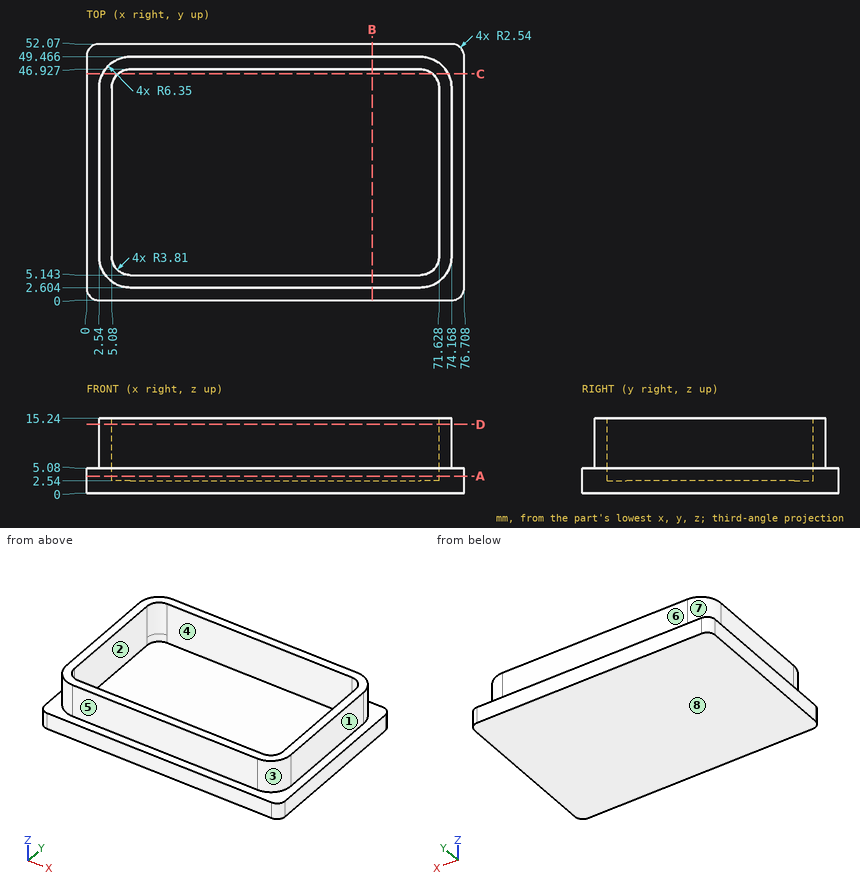
Drawing for the job (mm, zero at the part's lowest x, y, z). A direction names the side the tool comes from. Round coordinates to 2 decimals unless told otherwise and drop trailing zeros. Loops run counter-clockwise (first coordinate to the right, second up) from the corner with the lowest first, then second, coordinate; pieces in that order, holes last. Notation, with made-up numbers: M 11,68.25 L 17,68.25 A17 cw 17,99.25 Z; hole C -10,73 d1. An arc over 180 degrees is marked long. Use a Markdown table: item, result. Add a question column.
(1) Cut at A-A (z = 3.5). Give the cut face in (x, y), and give its area (3 significant figures).
(2) Flat gauge pins, fed straight in: pin 1 (4 mm diameter, centred on x = 20, z = 8.5, fed in from +Y); pin 2 (5 mm diameter, centred on y = 22.5, z = 10.5, fed in from +X); pin 3 (2 mm diameter, centred on x = 65, y = 16, fed in from +Z). Where does each tip first touch, or does it go through?
(3) Cut at B-B (x = 58). Give the cut face in (y, z).
(4) Cut at D-D (z = 14). Give the cut face in (x, y).
(5) Cut at C-C (y = 46). Give the cut face in (x, z) (1 decimal).
(6) Pull direction Y, two halves, no side cores. Call the marked faces 1, 2 and 3: +Y half, -Y half, draft (parallel to the pull), parting line (faces both ways), or undercut.
(7) Which spindle directions (+Z, -Z, +X, -X, +Y, -Y) get a long thin tool onto all of the face, cutting with end or side? Do the marked faces 4, 5, 6, 7 and 8. Say none if no direction does.
(8) Drill centre lines: line 1 (Y direction, x = 30, z = 5.75); line 2 (X direction, y = 25, z = 12.5); line 3 (X direction, y = 14, z = 3.5). Where is each one in solid material? Low to high.
Geometry says:
| question | item | result |
|---|---|---|
| 1 | outline | M 0,2.54 A2.54 ccw 2.54,0 L 74.17,0 A2.54 ccw 76.71,2.54 L 76.71,49.53 A2.54 ccw 74.17,52.07 L 2.54,52.07 A2.54 ccw 0,49.53 Z; hole M 5.08,8.95 A3.81 ccw 8.89,5.14 L 67.82,5.14 A3.81 ccw 71.63,8.95 L 71.63,43.12 A3.81 ccw 67.82,46.93 L 8.89,46.93 A3.81 ccw 5.08,43.12 Z |
| 1 | area | 1,220 mm² |
| 2 | pin 1 | stops at y = 49.47 |
| 2 | pin 2 | stops at x = 74.17 |
| 2 | pin 3 | stops at z = 2.54 |
| 3 | outline | M 0,0 L 52.07,0 L 52.07,5.08 L 49.47,5.08 L 49.47,15.24 L 46.93,15.24 L 46.93,2.54 L 5.14,2.54 L 5.14,15.24 L 2.6,15.24 L 2.6,5.08 L 0,5.08 Z |
| 4 | outline | M 2.54,8.95 A6.35 ccw 8.89,2.6 L 67.82,2.6 A6.35 ccw 74.17,8.95 L 74.17,43.12 A6.35 ccw 67.82,49.47 L 8.89,49.47 A6.35 ccw 2.54,43.12 Z; hole M 5.08,8.95 A3.81 ccw 8.89,5.14 L 67.82,5.14 A3.81 ccw 71.63,8.95 L 71.63,43.12 A3.81 ccw 67.82,46.93 L 8.89,46.93 A3.81 ccw 5.08,43.12 Z |
| 5 | outline | M 0,0 L 76.7,0 L 76.7,5.1 L 73.5,5.1 L 73.5,15.2 L 70.3,15.2 L 70.3,2.5 L 6.4,2.5 L 6.4,15.2 L 3.2,15.2 L 3.2,5.1 L 0,5.1 Z |
| 6 | face 1 | draft |
| 6 | face 2 | undercut |
| 6 | face 3 | -Y half |
| 7 | face 4 | +Z |
| 7 | face 5 | +Z, +X, -X, -Y |
| 7 | face 6 | +Z, +X, -X, +Y |
| 7 | face 7 | +Z, -X, +Y |
| 7 | face 8 | -Z, +X, -X, +Y, -Y |
| 8 | line 1 | y = 2.6 to 5.14, 46.93 to 49.47 |
| 8 | line 2 | x = 2.54 to 5.08, 71.63 to 74.17 |
| 8 | line 3 | x = 0 to 5.08, 71.63 to 76.71 |
